Part model, mm, in its own coordinate system. Face numbers are marked on the shaded views. A direction names the side the tool comes from. Round coordinates to 2 decimals unless told otherwise and drop trailing zeros. Loops run counter-clockwise (first coordinate to the right, second up) from the corner with the lowest first, then second, coordinate; pieces in that order, holes last. Notation, with made-up numbers: (52, 8) -> (81, 8) arc R22 cw to (81, 15) -> close; hole circle Ø1 at (31, 81.5). An arc over 180 degrees is marked (long way). Answer as a JSON object with one key per item and string values. Group by question number.
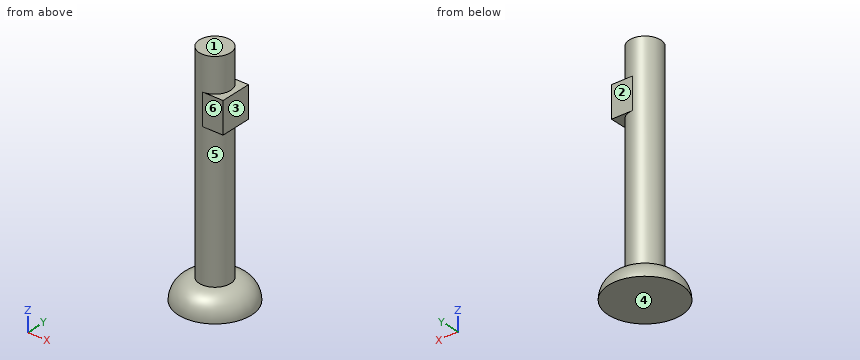
from build123d import *

# Parameters (mm, degrees)
F0_R     = 44.45
F1_DEPTH = 25.4
F2_R     = 25.39999
F3_DEPTH = 254
F4_W     = 38.1
F4_H     = 38.1
F5_DEPTH = 25.4


# Not quite as in the source:
# - a fillet or chamfer is up to 0.001 mm smaller than in the source, because OpenCascade refuses the exact size


with BuildPart() as f1:
    # F0 (on Top) → F1 (new body)
    with BuildSketch(Plane.XY):
        Circle(F0_R)
    extrude(amount=F1_DEPTH)

    # F2 (radius 25.4 in the source; OpenCascade refuses exactly that, so slightly less here)
    f2_edges = [f1.edges().sort_by_distance(p)[0] for p in [
        (-44.45, 0, 25.4),
    ]]
    fillet(f2_edges, radius=F2_R)

    # F3 (add): a face of the model
    f3_faces = [f1.faces().sort_by_distance(p)[0] for p in [
        (0, 0, 25.4),
    ]]
    extrude(f3_faces, amount=F3_DEPTH)

    # F4 (on Right) → F5 (join)
    with BuildSketch(Plane.YZ):
        with Locations((0, 218.8449014022)):
            Rectangle(F4_W, F4_H)
    extrude(amount=F5_DEPTH)


solid = f1.part
Item 1: Two-plate mould, pull along Z, no slides. Class the marked faces 4, 5 and 6: pulls with the +Z half, pulls with the -Z half, needs draft (parallel to the pull), parting line crosses it, or undercut.
Item 2: Which spindle directions (+Z, -Z, +X, -X, +Y, -Y) get a long thin tool onto all of the face, cutting with end or side? Do the marked faces 1, 2 and 3. Say none if no direction does.
Item 3: Band-saw the part on A-A, the plane z = 202.5. List the corners of the cut face in (x, y), plus the area to 3 significant figures.
Item 4: Drill centre lines: line 1 (X direction, y = -0.5, z = 261); line 2 (Y direction, x = 7, z = 236.5); line 3 (Z direction, x = 8.5, y = 29). Where is each one in solid material? Low to high.
Item 5: Drop flat-ended pins along their axis: pin 1 Ø1 at (x, y) = (18.5, 4.5) entering from -Z; pin 2 Ø1 at (x, y) = (30.5, 27) entering from +Z; pin 3 Ø5 at (x, z) = (-7, 204.5) entering from -Y; pin 4 Ø12.5 at (x, z) = (15.5, 215.5) entering from +Y. Give the stop position or say it passes through.
Entries:
{
 "1": {"face 4": "pulls with the -Z half", "face 5": "undercut", "face 6": "needs draft"},
 "2": {"face 1": "+Z, +X, -X, +Y, -Y", "face 2": "+Z, +X, -X, +Y", "face 3": "+Z, +X, +Y, -Y"},
 "3": {"outline": "(0.02, -19.05) -> (25.4, -19.05) -> (25.4, 19.05) -> (0.02, 19.05) arc R19.05 ccw to start", "area": "1,540 mm²"},
 "4": {"line 1": "-19.04 to 19.04", "line 2": "-19.05 to 19.05", "line 3": "0 to 22.81"},
 "5": {"pin 1": "z = 0", "pin 2": "z = 14.01", "pin 3": "y = -18.51", "pin 4": "y = 19.05"}
}
